```python
from build123d import *

# Parameters (mm, degrees)
SKETCH1_W               = 770
SKETCH1_H               = 470
BOSS_EXTRUDE1_DEPTH     = 1.5
CUT_EXTRUDE4_DEPTH      = 17
CUT_EXTRUDE4_DEPTH_BACK = 10
SKETCH3_W               = 316
SKETCH3_H               = 420


with BuildPart() as part:
    # Sketch1 → Boss-Extrude1 (new body)
    with BuildSketch(Plane.XY):
        Rectangle(SKETCH1_W, SKETCH1_H)
    extrude(amount=BOSS_EXTRUDE1_DEPTH)

    # Sketch3 → Cut-Extrude4 (cut, two sides: drawn at the far end of the back side and taken through both)
    with BuildSketch(Plane.XY.offset(1.5).offset(-CUT_EXTRUDE4_DEPTH_BACK)):
        Rectangle(SKETCH3_W, SKETCH3_H)
    extrude(amount=CUT_EXTRUDE4_DEPTH + CUT_EXTRUDE4_DEPTH_BACK, mode=Mode.SUBTRACT)


solid = part.part
```
Geometry: final body of the model. Coordinates: model frame, mm. Round coordinates to 2 decimals unless told otherwise and drop trailing zeros. Loops run counter-clockwise (first coordinate to the right, second up) from the corner with the lowest first, then second, coordinate; pieces in that order, holes last. Notation, with made-up numbers: (-40, -18.75) -> (-8, -18.75) arc R33 cw to (-8, 13.25) -> close; hole circle Ø3 at (28.5, -7). An arc over 180 degrees is marked (long way). Write each question's results on one line, items separated by ' | '.
Item 1: Cut plane B-B on y = -127. Return the cut outline in (x, z), and give its area (3 significant figures).
Answers below:
outline: (-385, 0) -> (-158, 0) -> (-158, 1.5) -> (-385, 1.5) -> close; (158, 0) -> (385, 0) -> (385, 1.5) -> (158, 1.5) -> close | area: 681 mm²
Item 2: Pin query (flat end, axial travel): pin 1 Ø10 at (x, y) = (-251, 41.5) entering from -Z. Return the tip coordinate at first contact, or that it passes through.
Answers below:
pin 1: stops at z = 0
Item 3: Cut plane A-A on x = -134. Return the cut outline in (y, z), and give its area (3 significant figures).
Answers below:
outline: (-235, 0) -> (-210, 0) -> (-210, 1.5) -> (-235, 1.5) -> close; (210, 0) -> (235, 0) -> (235, 1.5) -> (210, 1.5) -> close | area: 75.0 mm²
Item 4: Cut plane C-C on z = 1.2. Return the cut outline in (x, y), and give its area (3 significant figures).
Answers below:
outline: (-385, -235) -> (385, -235) -> (385, 235) -> (-385, 235) -> close; hole (-158, -210) -> (158, -210) -> (158, 210) -> (-158, 210) -> close | area: 229,000 mm²
Item 5: Line query: probe 1 along X at (y, z) = (40, 1.15); probe 2 along Y at (x, z) = (94.5, 1). Output: solid intervals per line, ascending. Write a range as [from, to].
Answers below:
probe 1: x = [-385, -158], [158, 385] | probe 2: y = [-235, -210], [210, 235]
